CAD build for the part. Positions are in the model's coordinates, mm. A direction names the side the tool comes from. Coordinates: 2 decimals unless noted, no trailing zeros. Loops run counter-clockwise (first coordinate to the right, second up) from the corner with the lowest first, then second, coordinate; pieces in that order, holes last. Notation, with made-up numbers: (-11, 57.25) - (47, 57.25) arc R22 cw to (47, 81.25) - close; hole circle Ø4 at (-8, -37.75). An arc over 180 degrees is marked (long way). Put each result on its own line as item: value.
Autodesk Inventor part; units mm, degrees
ref_plane "YZ Plane" through (0, 0, 0) normal (1, 0, 0) x (0, 1, 0)
ref_plane "XZ Plane" through (0, 0, 0) normal (0, 1, 0) x (-1, 0, 0)
ref_plane "XY Plane" through (0, 0, 0) normal (0, 0, 1) x (1, 0, 0)
sketch "Sketch1" plane through (0, 0, 0) normal (0, 1, 0) x (-1, 0, 0)
  line L0 (-8, 14) -> (8, 14)
  line L1 (8, 14) -> (8, -14)
  line L2 (8, -14) -> (-8, -14)
  line L3 (-8, -14) -> (-8, 14)
  line L4 (-8, 14) -> (8, -14) construction
  line L5 (8, 14) -> (-8, -14) construction
  point P0 (0, 0)
  dimension "d0" = 16
  dimension "d1" = 28
extrude "Extrusion1" add sketch "Sketch1" along normal mid plane 10
fillet "Fillet1" radius 2 4 edges at (8, 0, 14) (8, 0, -14) (-8, 0, 14) (-8, 0, -14)
sketch "Sketch2" plane through (0, 5, 0) normal (0, 1, 0) x (1, 0, 0)
  arc A0 (-6, 14) -> (-8, 12) centre (-6, 12) ccw
  line L0 (-8, 12) -> (-8, -12)
  arc A1 (-8, -12) -> (-6, -14) centre (-6, -12) ccw
  line L1 (-6, -14) -> (6, -14)
  arc A2 (6, -14) -> (8, -12) centre (6, -12) ccw
  line L2 (8, -12) -> (8, 12)
  arc A3 (8, 12) -> (6, 14) centre (6, 12) ccw
  line L3 (6, 14) -> (-6, 14)
  circle A4 centre (-5, 11) radius 1.5
  circle A5 centre (5, -11) radius 1.5
  point P0 (0, 0)
  dimension "d5" = 3
  dimension "d6" = 3
  dimension "d7" = 3
  dimension "d8" = 3
  dimension "d9" = 3
extrude "Extrusion2" cut sketch "Sketch2" against normal blind 10 contours A4 | A5
sketch "Sketch3" plane through (-6, -5, 14) normal (0, 0, 1) x (1, 0, 0)
  line L0 (0, 0) -> (0, 10)
  line L1 (12, 0) -> (0, 0)
  line L2 (12, 10) -> (12, 0)
  line L3 (0, 10) -> (12, 10)
  line L4 (3.2, 10) -> (4.1, 10)
  line L5 (4.1, 10) -> (4.1, 0)
  line L6 (4.1, 0) -> (3.2, 0)
  line L7 (3.2, 0) -> (3.2, 10)
  line L8 (8.8, 10) -> (7.9, 10)
  line L9 (7.9, 10) -> (7.9, 0)
  line L10 (7.9, 0) -> (8.8, 0)
  line L11 (8.8, 0) -> (8.8, 10)
  line L12 (1, 2) -> (11, 2)
  line L13 (11, 2) -> (11, 8) construction
  line L14 (11, 8) -> (1, 8)
  line L15 (1, 8) -> (1, 2) construction
  point P0 (6, 5)
  point P1 (8.8, 8)
  point P2 (7.9, 8)
  point P3 (7.9, 2)
  point P4 (8.8, 2)
  point P5 (4.1, 8)
  point P6 (3.2, 8)
  point P7 (3.2, 2)
  point P8 (4.1, 2)
  point P9 (11, 5)
  point P10 (12, 5)
  dimension "d12" = 0.9
  dimension "d14" = 10
  dimension "d15" = 6
extrude "Extrusion3" add sketch "Sketch3" along normal blind 9 contours L7 L14 L5 L12 | L9 L14 L11 L12
sketch "Sketch4" plane through (-2.8, -3, 14) normal (-1, 0, 0) x (0, 0, 1)
  line L0 (0, 0) -> (0, 6)
  line L1 (9, 6) -> (9, 0)
  circle A0 centre (6.0959, 3) radius 1
  line L2 (0, 0) -> (9, 0)
  line L3 (0, 6) -> (9, 6)
  point P0 (-14, 3)
  point P1 (9, 3)
  dimension "d18" = 2
extrude "Extrusion4" cut sketch "Sketch4" against normal through all contours A0
chamfer "Chamfer1" distance 2 angle 45 4 edges at (-2.35, 3, 23) (2.35, 3, 23) (2.35, -3, 23) (-2.35, -3, 23)
sketch "Sketch5" plane through (0, 0, 0) normal (0, 1, 0) x (-1, 0, 0)
  circle A0 centre (-5, 11) radius 1.5
  circle A1 centre (5, -11) radius 1.5
  arc A2 (6, -14) -> (8, -12) centre (6, -12) ccw
  line L0 (8, -12) -> (8, 12)
  arc A3 (8, 12) -> (6, 14) centre (6, 12) ccw
  line L1 (6, 14) -> (-6, 14)
  arc A4 (-6, 14) -> (-8, 12) centre (-6, 12) ccw
  line L2 (-8, 12) -> (-8, -12)
  arc A5 (-8, -12) -> (-6, -14) centre (-6, -12) ccw
  line L3 (-6, -14) -> (6, -14)
  line L4 (-8, 6.8206) -> (-9.5, 6.8206)
  line L5 (-9.5, 6.8206) -> (-12.7296, -23.9071)
  line L6 (-11.8345, -24.0012) -> (-8.6896, 5.9206)
  line L7 (-8.6896, 5.9206) -> (-8, 5.9206)
  line L8 (-11.8345, -24.0012) -> (-12.7296, -23.9071)
  line L9 (-12.7296, -23.9071) -> (-14.7187, -23.6981)
  line L10 (-14.7187, -23.6981) -> (-14.6555, -23.0969)
  line L11 (-14.6555, -23.0969) -> (-12.6664, -23.306)
  circle A6 centre (-14.6871, -23.3975) radius 2
  line L12 (-8, 12) -> (-8, -12)
  point P0 (0, 0)
  point P1 (-12.6893, -23.3036)
  point P2 (-12.7525, -23.9047)
  dimension "d24" = 0.9
  dimension "d25" = 4
  dimension "d26" = 2
  dimension "d27" = 6
  dimension "d28" = 1.5
extrude "Extrusion5" add sketch "Sketch5" along normal mid plane 4 contours L7 L6 L8 L5 L4 L2 | L5 A6 L11 | L9 A6 L5 | A6 L9 L10 L11 | L11 L10 L9 A6
sketch "Sketch6" plane through (0, 0, 0) normal (0, 1, 0) x (-1, 0, 0)
  line L0 (8, -12) -> (8, 12)
  line L1 (8, 1.4634) -> (12, 1.4634)
  line L2 (12, 1.4634) -> (12, 2.3634)
  line L3 (12, 2.3634) -> (8, 2.3634)
  line L4 (8, 2.3634) -> (8, 1.4634)
  line L5 (12, 2.3634) -> (11.1, 2.3634)
  line L6 (11.1, 2.3634) -> (11.1, 10.4634)
  line L7 (11.1, 10.4634) -> (12, 10.4634)
  line L8 (12, 10.4634) -> (12, 2.3634)
  point P0 (0, 0)
  dimension "d31" = 4
  dimension "d32" = 0.9
  dimension "d33" = 0.9
  dimension "d34" = 9
extrude "Extrusion6" add sketch "Sketch6" along normal mid plane 6
properties part number "FIN_DE_CARRERA" material "Steel, Mild, Welded"
Q1. Wall check: L1, parallel to Z at x = -5, y = 1.25; L2, parallel to X at y = 1.5, z = -11; L3, parallel to Z at x = 5, y = -2.5. Give the ranges that are in metal, low to high. Write a range as from..to.
Determined:
L1: -14..-12.5, -9.5..14
L2: -8..-6.5, -3.5..8, 10.47..11.37
L3: -14..9.5, 12.5..14
Q2. Slice it at C-C, the plane x = 4. Give the cut face in (y, z), then the cut area to 3 significant figures.
Determined:
outline: (-5, -14) - (5, -14) - (5, 9.88) - (-5, 9.88) - close; (-5, 12.12) - (5, 12.12) - (5, 14) - (-5, 14) - close
area: 258 mm2
Q3. Mould opens along X. For faces 4 (the cylindrical face through (-7.4, -0.07, 13.43)), 5 (the cylindrical face through (2.344, 0.044, 19.097)), 6 (the flat face through (-1.9, 0, 18)) say: +X half, -X half, draft (parallel to the pull), parting line (faces both ways), or undercut.
Determined:
face 4: -X half
face 5: draft
face 6: undercut
Q4. Slice it at D-D, the plane y = 0. State how many separate pieces and enclosed holes the cut face has, then the cut area to 3 significant figures.
Determined:
separate pieces: 3
enclosed holes: 2
area: 495 mm2
Q5. Tool access for faces 1 (the flat face through (-11.3, -3, 5)), 2 (the flat face through (1.9, 0, 18)), 3 (the flat face through (2.3, -3, 17.5)): list every direction of +Z, -Z, +X, -X, +Y, -Y with a clear straight run to the whole face (end or side of a thin tool).
Determined:
face 1: +Z, -Z, -X, -Y
face 2: +Z, +Y, -Y
face 3: +Z, +X, -X, -Y
Q6. Slice it at A-A, the plane z = 11. Give the cut face in (x, y).
Determined:
outline: (-8, -5) - (3.5, -5) - (3.5, 5) - (-8, 5) - close; (6.5, -5) - (8, -5) - (8, 5) - (6.5, 5) - close
Q7. Pin check, flat tips, straight feed: pin 1 Ø1.8 at (y, z) = (1, 5.5) entering from +X; pin 2 Ø3 at (y, z) = (1, -2) entering from +X; pin 3 Ø1 at (x, z) = (-2, 18.5) entering from -Y. Stop position of each tip, or through.
Determined:
pin 1: x = 9.73
pin 2: x = 10.58
pin 3: y = -3
Q8. Slice it at B-B, the plane y = -2.5. Give the cut face in (x, z).
Determined:
outline: (-12, 1.46) - (-8, 1.46) - (-8, -12) arc R2 ccw to (-6, -14) - (6, -14) arc R2 ccw to (8, -12) - (8, 12) arc R2 ccw to (6, 14) - (2.8, 14) - (2.8, 21.5) - (1.9, 21.5) - (1.9, 14) - (-1.9, 14) - (-1.9, 21.5) - (-2.8, 21.5) - (-2.8, 14) - (-6, 14) arc R2 ccw to (-8, 12) - (-8, 2.36) - (-11.1, 2.36) - (-11.1, 10.46) - (-12, 10.46) - close; hole circle Ø3 at (-5, -11); hole circle Ø3 at (5, 11)
